The model under review builds one solid part; all positions refer to its coordinate system, in mm. A direction names the side the tool comes from. Coordinates: 2 decimals unless noted, no trailing zeros. Order: outer loops, then holes, each group sorted by start corner. A loop starts at its lowest first (then second) coordinate and runs counter-clockwise, first axis right, second up. Notation, with made-up numbers: M 6,20 L 19,20 A9 ccw 19,28 Z; hole C 63.25,-38 d1. An arc over 180 degrees is marked long. Write each question's results on one line, items separated by ' | '.
Autodesk Inventor part; units mm, degrees
ref_plane "YZ Plane" through (0, 0, 0) normal (1, 0, 0) x (0, 1, 0)
ref_plane "XZ Plane" through (0, 0, 0) normal (0, 1, 0) x (-1, 0, 0)
ref_plane "XY Plane" through (0, 0, 0) normal (0, 0, 1) x (1, 0, 0)
sketch "Sketch5" plane through (0, 0, 0) normal (0, 1, 0) x (-1, 0, 0)
  circle A0 centre (0, 0) radius 11
  circle A1 centre (0, 0) radius 14
  dimension "d11" = 22
  dimension "d12" = 3
extrude "Extrusion4" add sketch "Sketch5" along normal blind 19.225
sketch "Sketch6" plane through (0, 0, 0) normal (0, -1, 0) x (1, 0, 0)
  circle A0 centre (0, 0) radius 14
extrude "Extrusion5" add sketch "Sketch6" along normal blind 3
fillet "Fillet2" radius 3 1 edges at (-14, -3, 0)
properties part number "Cap"
1) Take a section at D-D on y = -0.75. State the section outline as (x, z) points.
Solutions:
outline: C 0,0 d27.81
2) Take a section at A-A on x = 0. State the section outline as (y, z) points (1 decimal).
Solutions:
outline: M -3,-11 A3 ccw 0,-14 L 19.2,-14 L 19.2,-11 L 0,-11 L 0,11 L 19.2,11 L 19.2,14 L 0,14 A3 ccw -3,11 Z
3) To check wall thickness, follow line 1 along Z through (x, y) = (0, 8.5); line 2 along Y through (x, z) = (9.5, -0.5); line 3 along X through (y, z) = (14.5, -1). State the ranges of each line that lie inside material, in increasing order.
Solutions:
line 1: -14 to -11, 11 to 14 | line 2: -3 to 0 | line 3: -13.96 to -10.95, 10.95 to 13.96
4) The part is to be moulded in two halves that separate along Z. For faces 3 (the flat face through (-6.2, 19.225, -9.3)), 4 (the cylindrical face through (2.38, 9.48, 10.74)), say which applies: pulls with the +Z half, pulls with the -Z half, needs draft (parallel to the pull), parting line crosses it, or undercut.
Solutions:
face 3: needs draft | face 4: undercut
5) For pin 1 (1.5 mm diameter, centred on x = 4, y = 3, fed in from -Z); pin 2 (8 mm diameter, centred on x = -6.5, y = 7, fed in from +Z) (3 decimals); pin 3 (13 mm diameter, centred on x = 0, z = 0, fed in from +Y), all flat-tipped, find the tip position at first contact; note any pin that passes through.
Solutions:
pin 1: z = -13.62 | pin 2: z = 13.775 | pin 3: y = 0
6) Take a section at B-B on z = 0. State the section outline as (x, y) points (1 decimal).
Solutions:
outline: M -14,0 A3 ccw -11,-3 L 11,-3 A3 ccw 14,0 L 14,19.2 L 11,19.2 L 11,0 L -11,0 L -11,19.2 L -14,19.2 Z
7) For faces 1 (the flat face through (0, 0, 0)), 2 (the flat face through (0, -3, 0)), list the 3-axis set-ups (+Z, -Z, +X, -X, +Y, -Y) from which the entire face can be reached by the end or side of a thin tool; tool diameter is ignored.
Solutions:
face 1: +Y | face 2: +Z, -Z, +X, -X, -Y
8) Take a section at C-C on y = 13. State the section outline as (x, z) points, plus the area to 3 significant figures.
Solutions:
outline: C 0,0 d28; hole C 0,0 d22 | area: 236 mm2
